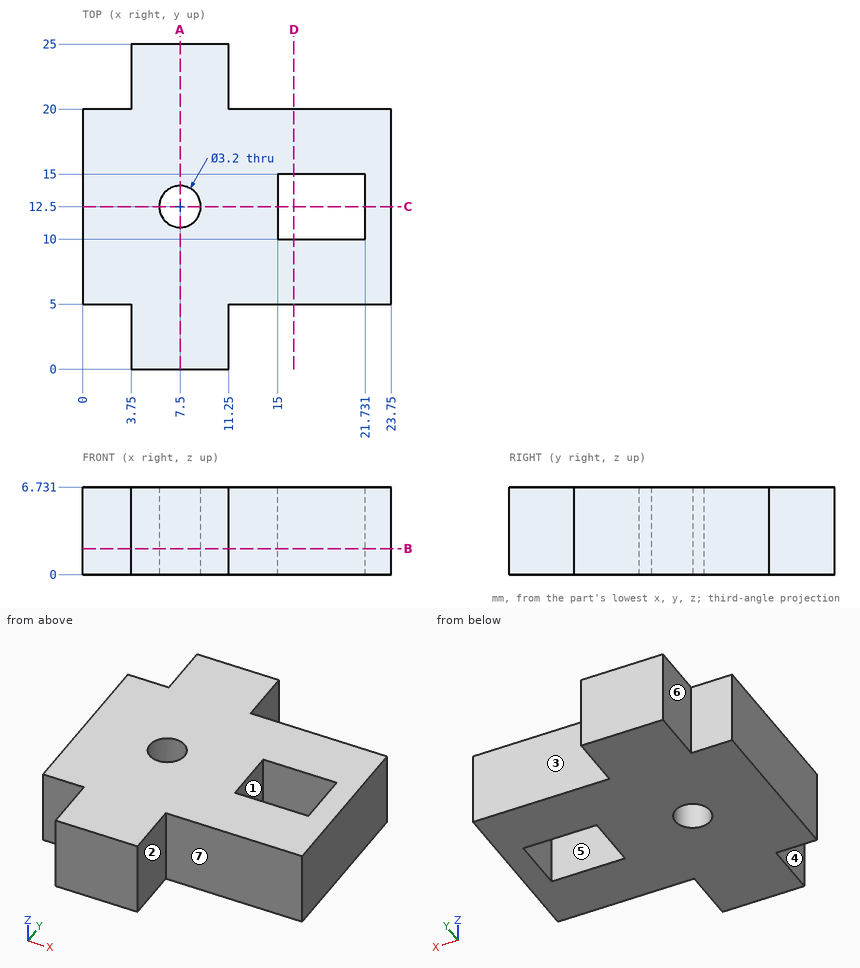
Here's the drawing with two shaded views (mm, measured from the low corner). I have some questions. A direction names the side the tool comes from. Coordinates: 2 decimals unless noted, no trailing zeros. Write each loop counter-clockwise with the first axis right and the second up, starting at its lowest first coordinate (ties: lowest second). Pieces come first, ordered by that corner, then holes. Notation, with made-up numbers: M -28,7.25 L -1,7.25 A20 cw -1,35.25 Z; hole C 10.5,-17 d4. An arc over 180 degrees is marked long. Answer as CSV lines item,"result".
Item 1: We'd pull the mould along X, two halves only. Please class the marked faces 5, 6 and 7: +X half, -X half, draft (parallel to the pull), parting line (faces both ways), or undercut.
Geometry results:
face 5,"undercut"
face 6,"-X half"
face 7,"draft"
Item 2: Imagine slicing it at B-B on z = 2. List the corners of the cut face in (x, y) for me.
Geometry results:
outline,"M 0,5 L 3.75,5 L 3.75,0 L 11.25,0 L 11.25,5 L 23.75,5 L 23.75,20 L 11.25,20 L 11.25,25 L 3.75,25 L 3.75,20 L 0,20 Z; hole C 7.5,12.5 d3.2; hole M 15,10 L 21.73,10 L 21.73,15 L 15,15 Z"
Item 3: Imagine slicing it at D-D on x = 16.25. List the corners of the cut face in (y, z) for me.
Geometry results:
outline,"M 5,0 L 10,0 L 10,6.73 L 5,6.73 Z; M 15,0 L 20,0 L 20,6.73 L 15,6.73 Z"
Item 4: Imagine slicing it at A-A on x = 7.5. List the corners of the cut face in (y, z) for me, plus the area to 3 significant figures.
Geometry results:
outline,"M 0,0 L 10.9,0 L 10.9,6.73 L 0,6.73 Z; M 14.1,0 L 25,0 L 25,6.73 L 14.1,6.73 Z"
area,"147 mm2"
Item 5: I'm going to push flat-ended pins straight in: P1, Ø3.5, axis at x = 20, z = 2.5, coming from the +Y side; P2, Ø3.5, axis at x = 17, z = 2.5, coming from the -Y side; P3, Ø2.5, axis at x = 7.5, y = 12.5, coming from the +Z side; P4, Ø2.5, axis at y = 3, z = 2.5, coming from the -X side. Where does each tip first touch, or does it pass through?
Geometry results:
P1,"stops at y = 20"
P2,"stops at y = 5"
P3,"passes through"
P4,"stops at x = 3.75"
Item 6: Imagine slicing it at C-C on y = 12.5. List the corners of the cut face in (x, z) for me, plus the area to 3 significant figures.
Geometry results:
outline,"M 0,0 L 5.9,0 L 5.9,6.73 L 0,6.73 Z; M 9.1,0 L 15,0 L 15,6.73 L 9.1,6.73 Z; M 21.73,0 L 23.75,0 L 23.75,6.73 L 21.73,6.73 Z"
area,"93.0 mm2"
Item 7: On a 3-axis mill with a long thin cutter (end or side, diameter ignored), from which of +Z, -Z, +X, -X, +Y, -Y can I reach the whole of each face in a straight line? I mean the marked faces 1, 2, 3 and 4. Say none if no direction works.
Geometry results:
face 1,"+Z, -Z"
face 2,"+Z, -Z, +X, -Y"
face 3,"+Z, -Z, +X, +Y"
face 4,"+Z, -Z, -X, -Y"
Item 8: Please list where these lines run through material, in increasing order: line 1 along Y through (x, z) = (7.5, 5.5); line 2 along Y through (x, z) = (21.25, 6.25); line 3 along Y through (x, z) = (2, 5.75).
Geometry results:
line 1,"y = 0 to 10.9, 14.1 to 25"
line 2,"y = 5 to 10, 15 to 20"
line 3,"y = 5 to 20"
